from build123d import *

# Parameters (mm, degrees)
SKETCH1_R           = 15.5
SKETCH1_R_2         = 1.75
BOSS_EXTRUDE1_DEPTH = 16
SKETCH2_R           = 18.5
SKETCH2_R_2         = 1.75
BOSS_EXTRUDE2_DEPTH = 4
BOSS_EXTRUDE3_START = 4
SKETCH3_R           = 18.5
SKETCH3_R_2         = 1.75
BOSS_EXTRUDE3_DEPTH = 4
FILLET1_R           = 5
CHAMFER1_SIZE       = 1


with BuildPart() as part:
    # Sketch1 → Boss-Extrude1 (new body)
    with BuildSketch(Plane(origin=(0, 0, 0), x_dir=(1, 0, 0), z_dir=(0, 1, 0))):
        with Locations(Location((0, 0, 0), (0, 0, 270))):
            Circle(SKETCH1_R)
        with Locations(Location((0, 0, 0), (0, 0, 270))):
            Circle(SKETCH1_R_2, mode=Mode.SUBTRACT)
    extrude(amount=BOSS_EXTRUDE1_DEPTH)

    # Sketch2 → Boss-Extrude2 (add)
    with BuildSketch(Plane(origin=(0, 16, 0), x_dir=(1, 0, 0), z_dir=(0, 1, 0))):
        with Locations(Location((0, 0, 0), (0, 0, 270))):
            Circle(SKETCH2_R)
        with Locations(Location((0, 0, 0), (0, 0, 270))):
            Circle(SKETCH2_R_2, mode=Mode.SUBTRACT)
    extrude(amount=BOSS_EXTRUDE2_DEPTH)

    # Sketch3 → Boss-Extrude3 (add)
    with BuildSketch(Plane.XZ.offset(BOSS_EXTRUDE3_START)):
        with Locations(Location((0, 0, 0), (0, 0, 90))):
            Circle(SKETCH3_R)
        with Locations(Location((0, 0, 0), (0, 0, 270))):
            Circle(SKETCH3_R_2, mode=Mode.SUBTRACT)
    extrude(amount=-BOSS_EXTRUDE3_DEPTH)

    # Fillet1
    # the kernel refuses this fillet: 5 mm, written as the material it takes off along each edge
    with BuildSketch(Plane(origin=(0, 20, 0), x_dir=(0, 0, 1), z_dir=(-1, 0, 0))) as fillet1_piece_1:
        with BuildLine():
            CenterArc((1.75 + FILLET1_R, -FILLET1_R), FILLET1_R, 90, 90)
            Line((1.75, -FILLET1_R), (1.75, 0))
            Line((1.75, 0), (1.75 + FILLET1_R, 0))
        make_face()
    revolve(axis=Axis((0, 20, 0), (0, 1, 0)), mode=Mode.SUBTRACT)
    with BuildSketch(Plane(origin=(0, -4, 0), x_dir=(0, 0, -1), z_dir=(-1, 0, 0))) as fillet1_piece_2:
        with BuildLine():
            CenterArc((1.75 + FILLET1_R, -FILLET1_R), FILLET1_R, 90, 90)
            Line((1.75, -FILLET1_R), (1.75, 0))
            Line((1.75, 0), (1.75 + FILLET1_R, 0))
        make_face()
    revolve(axis=Axis((0, -4, 0), (0, -1, 0)), mode=Mode.SUBTRACT)

    # Chamfer1
    chamfer1_edges = [part.edges().sort_by_distance(p)[0] for p in [
        (0, 0, -15.5),
        (0, 16, -15.5),
    ]]
    chamfer(chamfer1_edges, length=CHAMFER1_SIZE)


solid = part.part
The listing builds one solid part. Answer for the finished solid, in the listing's coordinates (mm). A direction names the side the tool comes from. Give positions to 0.01 mm unless a question says otherwise; leave off trailing zeros. Write each loop counter-clockwise with the first axis right and the second up, starting at its lowest first coordinate (ties: lowest second). Pieces come first, ordered by that corner, then holes. Notation, with made-up numbers: (29.5, 83.25) -> (54.5, 83.25) arc R28 cw to (54.5, 117.25) -> close; hole circle Ø11 at (56.25, 66). An arc over 180 degrees is marked (long way). Use a Markdown table: item, result.
(1) Section C-C, the plane y = 2 is taken. Determine the outline of the cut face in (x, z).
Return value:
| item | result |
|---|---|
| outline | circle Ø31 at (0, 0); hole circle Ø3.5 at (0, 0) |
(2) Determine the mould class of faces 1 (the flat face through (0, 20, 8)), 2 (the cylindrical face through (-7.086, 17.972, 17.089)), 3 (the flat face through (0, 16, -17)) for opening direction Y: released by +Y, released by -Y, zero draft, split by the parting line, or undercut.
Return value:
| item | result |
|---|---|
| face 1 | released by +Y |
| face 2 | zero draft |
| face 3 | undercut |
(3) Section B-B, the plane x = 0 is taken. Determine the outline of the cut face in (y, z), then the cut area to 3 significant figures.
Return value:
| item | result |
|---|---|
| outline | (-4, -18.5) -> (0, -18.5) -> (0, -16.5) -> (1, -15.5) -> (15, -15.5) -> (16, -16.5) -> (16, -18.5) -> (20, -18.5) -> (20, -6.75) arc R5 ccw to (15, -1.75) -> (1, -1.75) arc R5 ccw to (-4, -6.75) -> close; (-4, 6.75) arc R5 ccw to (1, 1.75) -> (15, 1.75) arc R5 ccw to (20, 6.75) -> (20, 18.5) -> (16, 18.5) -> (16, 16.5) -> (15, 15.5) -> (1, 15.5) -> (0, 16.5) -> (0, 18.5) -> (-4, 18.5) -> close |
| area | 689 mm2 |
(4) For faces 4 (the cylindrical face through (15.368, 7.902, -2.018)), 5 (the flat face through (0, -4, 8)), determine the directions among +Z, -Z, +X, -X, +Y, -Y from which every point of the face is accessible in a straight line to the end or side of a thin tool.
Return value:
| item | result |
|---|---|
| face 4 | none |
| face 5 | +Z, -Z, +X, -X, -Y |
(5) Flat-ended cylindrical pins translate along their axes: P1, Ø5, axis at y = 3.5, z = -11.5, coming from the -X side; P2, Ø1.5, axis at y = 8.5, z = 9.5, coming from the -X side; P3, Ø8, axis at x = 7.5, y = 8.5, coming from the -Z side; P4, Ø5, axis at x = -1, y = 15, coming from the +Z side. Find the tip coordinate at first contact, or state that the pin passes through.
Return value:
| item | result |
|---|---|
| P1 | x = -12.62 |
| P2 | x = -12.79 |
| P3 | z = -15.1 |
| P4 | z = 18.5 |
(6) Find the intervals of material crossed by probe 1 along Y at (x, z) = (14, 9); probe 2 along Y at (x, z) = (-11, -12); probe 3 along X at (y, z) = (-1, 1.5), in increasing order. Write a range as from..to.
Return value:
| item | result |
|---|---|
| probe 1 | -4..0, 16..20 |
| probe 2 | -4..0.22, 15.78..20 |
| probe 3 | -18.44..-1.56, 1.56..18.44 |
(7) Section A-A, the plane z = 0 is taken. Determine the outline of the cut face in (x, y).
Return value:
| item | result |
|---|---|
| outline | (-18.5, -4) -> (-6.75, -4) arc R5 ccw to (-1.75, 1) -> (-1.75, 15) arc R5 ccw to (-6.75, 20) -> (-18.5, 20) -> (-18.5, 16) -> (-16.5, 16) -> (-15.5, 15) -> (-15.5, 1) -> (-16.5, 0) -> (-18.5, 0) -> close; (1.75, 1) arc R5 ccw to (6.75, -4) -> (18.5, -4) -> (18.5, 0) -> (16.5, 0) -> (15.5, 1) -> (15.5, 15) -> (16.5, 16) -> (18.5, 16) -> (18.5, 20) -> (6.75, 20) arc R5 ccw to (1.75, 15) -> close |
